Can you work these out from the model? Positions are in its coordinate system, mm. A direction names the side the tool comes from. Round coordinates to 2 decimals unless told otherwise and drop trailing zeros. Order: outer loops, then holes, each group sorted by start corner. A loop starts at its lowest first (then second) coordinate and runs counter-clockwise, first axis right, second up. Notation, with made-up numbers: M 58,86 L 105,86 A10 cw 105,96 Z; hole C 6,49 d2. An arc over 180 degrees is marked long. One line per question, with ' | ' between items.
```python
from build123d import *

# Parameters (mm, degrees)
SKETCH1_R           = 13.5
BOSS_EXTRUDE1_DEPTH = 4
CUT_EXTRUDE1_REACH  = 21.506
SKETCH2_R           = 3.25


with BuildPart() as part:
    # Sketch1 → Boss-Extrude1 (new body)
    with BuildSketch(Plane(origin=(0, 0, 0), x_dir=(1, 0, 0), z_dir=(0, 1, 0))):
        with Locations(Location((0, 0, 0), (0, 0, 270))):
            Circle(SKETCH1_R)
    extrude(amount=BOSS_EXTRUDE1_DEPTH)

    # Sketch2 → Cut-Extrude1 (cut, up to next)
    with BuildSketch(Plane(origin=(0, 4, 0), x_dir=(1, 0, 0), z_dir=(0, 1, 0)), mode=Mode.PRIVATE) as cut_extrude1_sk1:
        with BuildLine():
            Line((-9.337424698, -1.75), (-8, -1.75))
            ThreePointArc((-8, -1.75), (-6.25, 0), (-8, 1.75))
            Line((-8, 1.75), (-9.337424698, 1.75))
            ThreePointArc((-9.337424698, 1.75), (-9.338120985, 1.746280755), (-9.338815789, 1.742561233))
            ThreePointArc((-9.338815789, 1.742561233), (-11.25, 0), (-9.338815789, -1.742561233))
            ThreePointArc((-9.338815789, -1.742561233), (-9.338120985, -1.746280755), (-9.337424698, -1.75))
        make_face()
    cut_extrude1_tool1 = extrude(cut_extrude1_sk1.sketch, amount=-CUT_EXTRUDE1_REACH, mode=Mode.PRIVATE) & part.part
    # Sketch2 → Cut-Extrude1 (cut, up to next)
    with BuildSketch(Plane(origin=(0, 4, 0), x_dir=(1, 0, 0), z_dir=(0, 1, 0)), mode=Mode.PRIVATE) as cut_extrude1_sk2:
        with BuildLine():
            ThreePointArc((1.75, 9.337424698), (1.746280755, 9.338120985), (1.742561233, 9.338815789))
            ThreePointArc((1.742561233, 9.338815789), (0, 11.25), (-1.742561233, 9.338815789))
            ThreePointArc((-1.742561233, 9.338815789), (-1.746280755, 9.338120985), (-1.75, 9.337424698))
            Line((-1.75, 9.337424698), (-1.75, 8))
            ThreePointArc((-1.75, 8), (0, 6.25), (1.75, 8))
            Line((1.75, 8), (1.75, 9.337424698))
        make_face()
    cut_extrude1_tool2 = extrude(cut_extrude1_sk2.sketch, amount=-CUT_EXTRUDE1_REACH, mode=Mode.PRIVATE) & part.part
    # Sketch2 → Cut-Extrude1 (cut, up to next)
    with BuildSketch(Plane(origin=(0, 4, 0), x_dir=(1, 0, 0), z_dir=(0, 1, 0)), mode=Mode.PRIVATE) as cut_extrude1_sk3:
        with BuildLine():
            ThreePointArc((-1.742561233, -9.338815789), (0, -11.25), (1.742561233, -9.338815789))
            ThreePointArc((1.742561233, -9.338815789), (1.746280755, -9.338120985), (1.75, -9.337424698))
            Line((1.75, -9.337424698), (1.75, -8))
            ThreePointArc((1.75, -8), (0, -6.25), (-1.75, -8))
            Line((-1.75, -8), (-1.75, -9.337424698))
            ThreePointArc((-1.75, -9.337424698), (-1.746280755, -9.338120985), (-1.742561233, -9.338815789))
        make_face()
    cut_extrude1_tool3 = extrude(cut_extrude1_sk3.sketch, amount=-CUT_EXTRUDE1_REACH, mode=Mode.PRIVATE) & part.part
    # Sketch2 → Cut-Extrude1 (cut, up to next)
    with BuildSketch(Plane(origin=(0, 4, 0), x_dir=(1, 0, 0), z_dir=(0, 1, 0)), mode=Mode.PRIVATE) as cut_extrude1_sk4:
        with BuildLine():
            ThreePointArc((9.337424698, -1.75), (9.338120985, -1.746280755), (9.338815789, -1.742561233))
            ThreePointArc((9.338815789, -1.742561233), (11.25, 0), (9.338815789, 1.742561233))
            ThreePointArc((9.338815789, 1.742561233), (9.338120985, 1.746280755), (9.337424698, 1.75))
            Line((9.337424698, 1.75), (8, 1.75))
            ThreePointArc((8, 1.75), (6.25, 0), (8, -1.75))
            Line((8, -1.75), (9.337424698, -1.75))
        make_face()
    cut_extrude1_tool4 = extrude(cut_extrude1_sk4.sketch, amount=-CUT_EXTRUDE1_REACH, mode=Mode.PRIVATE) & part.part
    # Sketch2 → Cut-Extrude1 (cut, up to next)
    with BuildSketch(Plane(origin=(0, 4, 0), x_dir=(1, 0, 0), z_dir=(0, 1, 0)), mode=Mode.PRIVATE) as cut_extrude1_sk5:
        with Locations(Location((0, 0, 0), (0, 0, 270))):
            Circle(SKETCH2_R)
    cut_extrude1_tool5 = extrude(cut_extrude1_sk5.sketch, amount=-CUT_EXTRUDE1_REACH, mode=Mode.PRIVATE) & part.part
    add(cut_extrude1_tool1.solids().sort_by_distance((-8.749966, 4, 0))[0], mode=Mode.SUBTRACT)
    add(cut_extrude1_tool2.solids().sort_by_distance((0, 4, -8.749966))[0], mode=Mode.SUBTRACT)
    add(cut_extrude1_tool3.solids().sort_by_distance((0, 4, 8.749966))[0], mode=Mode.SUBTRACT)
    add(cut_extrude1_tool4.solids().sort_by_distance((8.749966, 4, 0))[0], mode=Mode.SUBTRACT)
    add(cut_extrude1_tool5.solids().sort_by_distance((0, 4, 0))[0], mode=Mode.SUBTRACT)


solid = part.part
```
(1) On a 3-axis mill with a long thin cutter (end or side, diameter ignored), from which of +Z, -Z, +X, -X, +Y, -Y can I reach the whole of each face in a straight line? I mean faces 1 (the flat face through (-3, 0, 3)), 2 (the flat face through (9, 2, 1.75)). Say none if no direction works.
Final values:
face 1: +Z, -Z, +X, -X, -Y | face 2: +Y, -Y
(2) If we section it at B-B on z = 7: Please give me the cut outline in (x, y), plus the area to 3 significant figures.
Final values:
outline: M -11.54,0 L -1.44,0 L -1.44,4 L -11.54,4 Z; M 1.44,0 L 11.54,0 L 11.54,4 L 1.44,4 Z | area: 80.9 mm^2
(3) If we section it at D-D on x = 11.75: Please give me the cut outline in (y, z).
Final values:
outline: M 0,-6.65 L 4,-6.65 L 4,6.65 L 0,6.65 Z
(4) If we section it at C-C on y = 1.7: State how many separate pieces and enclosed holes the cut face has, plus the area to 3 significant figures.
Final values:
separate pieces: 1 | enclosed holes: 5 | area: 480 mm^2
(5) Thinking about a two-plate mould opening in Z: for faces 3 (the cylindrical face through (-0.04, 2.03, 11.25)), 4 (the flat face through (-3, 4, 3)), which applies, released by +Z, released by -Z, zero draft, split by the parting line, or undercut?
Final values:
face 3: undercut | face 4: zero draft
(6) Will these pins go through, and if not, where does the flat tip stop? pin 1 Ø5.5 at (x, z) = (9.5, 0) entering from -Y; pin 2 Ø5 at (x, z) = (0, 0) entering from +Y; pin 3 Ø0.7 at (x, y) = (9, 1.5) entering from -Z; pin 4 Ø1.1 at (y, z) = (1, 8.5) entering from +X.
Final values:
pin 1: y = 0 | pin 2: through | pin 3: z = -10.36 | pin 4: x = 10.91
(7) Please list where these lines run through material, in increasing order: probe 1 along X at (y, z) = (1.5, 0); probe 2 along Z at (x, y) = (-1.5, 2.9); probe 3 along Z at (x, y) = (-7.75, 0.25). Write a range as [from, to].
Final values:
probe 1: [-13.5, -11.25], [-6.25, -3.25], [3.25, 6.25], [11.25, 13.5] | probe 2: [-13.42, -10.4], [-7.1, -2.88], [2.88, 7.1], [10.4, 13.42] | probe 3: [-11.05, -1.73], [1.73, 11.05]
(8) If we section it at A-A on x = 0: Please give me the cut outline in (y, z), plus the area to 3 significant figures.
Final values:
outline: M 0,-13.5 L 4,-13.5 L 4,-11.25 L 0,-11.25 Z; M 0,-6.25 L 4,-6.25 L 4,-3.25 L 0,-3.25 Z; M 0,3.25 L 4,3.25 L 4,6.25 L 0,6.25 Z; M 0,11.25 L 4,11.25 L 4,13.5 L 0,13.5 Z | area: 42.0 mm^2
